Autodesk Inventor part; units mm, degrees
ref_plane "YZ Plane" through (0, 0, 0) normal (1, 0, 0) x (0, 1, 0)
ref_plane "XZ Plane" through (0, 0, 0) normal (0, 1, 0) x (-1, 0, 0)
ref_plane "XY Plane" through (0, 0, 0) normal (0, 0, 1) x (1, 0, 0)
sketch "Sketch1" plane through (0, 0, 0) normal (0, 0, 1) x (1, 0, 0)
  line L0 (-15.875, 29.0994) -> (-12.7, 29.0994) construction
  line L1 (-15.875, 51.3244) -> (-15.875, 29.0994) construction
  arc A0 (-9.525, 57.6744) -> (-15.875, 51.3244) centre (-9.525, 51.3244) ccw construction
  line L2 (9.525, 57.6744) -> (-9.525, 57.6744) construction
  arc A1 (15.875, 51.3244) -> (9.525, 57.6744) centre (9.525, 51.3244) ccw construction
  line L3 (15.875, 29.0994) -> (15.875, 51.3244) construction
  line L4 (12.7, 29.0994) -> (15.875, 29.0994) construction
  line L5 (12.7, 51.3244) -> (12.7, 29.0994) construction
  arc A2 (12.7, 51.3244) -> (9.525, 54.4994) centre (9.525, 51.3244) ccw construction
  line L6 (-9.525, 54.4994) -> (9.525, 54.4994) construction
  arc A3 (-9.525, 54.4994) -> (-12.7, 51.3244) centre (-9.525, 51.3244) ccw construction
  line L7 (-12.7, 29.0994) -> (-12.7, 51.3244) construction
  line L8 (-30.0912, 10.1284) -> (-15.5432, 53.35)
  line L9 (30.0912, 10.1284) -> (15.5432, 53.35)
  arc A4 (-9.525, 57.6744) -> (-15.5432, 53.35) centre (-9.525, 51.3244) ccw
  arc A5 (15.5432, 53.35) -> (9.525, 57.6744) centre (9.525, 51.3244) ccw
  line L10 (-9.525, 57.6744) -> (9.525, 57.6744)
  arc A6 (-30.0912, 10.1284) -> (30.0912, 10.1284) centre (0, 0) ccw
  line L11 (-17.9505, 54.1603) -> (-32.4985, 10.9386)
  arc A7 (-32.4985, 10.9386) -> (32.4985, 10.9386) centre (0, 0) ccw
  line L12 (32.4985, 10.9386) -> (17.9505, 54.1603)
  arc A8 (17.9505, 54.1603) -> (9.525, 60.2144) centre (9.525, 51.3244) ccw
  line L13 (9.525, 60.2144) -> (-9.525, 60.2144)
  arc A9 (-9.525, 60.2144) -> (-17.9505, 54.1603) centre (-9.525, 51.3244) ccw
  circle A10 centre (0, 0) radius 31.75 construction
  dimension "d0" = 2.54
extrude "Extrusion1" add sketch "Sketch1" along normal blind 9.297
properties part number "Weight Shifter Tension Strap 2" material "Rubber"
Build history of the part. All positions in model axes, mm. A direction names the side the tool comes from. Coordinates: 2 decimals unless noted, no trailing zeros. Order: outer loops, then holes, each group sorted by start corner. A loop starts at its lowest first (then second) coordinate and runs counter-clockwise, first axis right, second up. Notation, with made-up numbers: (-17.75, 39.25) - (-1.75, 39.25) arc R26 ccw to (-1.75, 73.25) - close; hole circle Ø6 at (17.5, 76). An arc over 180 degrees is marked (long way). Put each result on its own line as item: value.
1. Saw through at A-A (x = 0). Write the cut outline in (y, z), and give its area (3 significant figures).
Answer sheet:
outline: (-34.29, 0) - (-31.75, 0) - (-31.75, 9.3) - (-34.29, 9.3) - close; (57.67, 0) - (60.21, 0) - (60.21, 9.3) - (57.67, 9.3) - close
area: 47.2 mm^2
2. Drop flat-ended pins along their axis: P1, Ø1.5, axis at y = 38.5, z = 8.5, coming from the +X side; P2, Ø10, axis at x = 9.5, y = -21.5, coming from the +Z side; P3, Ø5, axis at x = -14, z = 5.5, coming from the -Y side; P4, Ø4, axis at y = 3, z = 6, coming from the -X side. Give the stop position or say it passes through.
Answer sheet:
P1: stops at x = 23.47
P2: passes through
P3: stops at y = -32.3
P4: stops at x = -34.28
3. Saw through at C-C (y = 0). Write the cut outline in (x, z), and give its area (3 significant figures).
Answer sheet:
outline: (-34.29, 0) - (-31.75, 0) - (-31.75, 9.3) - (-34.29, 9.3) - close; (31.75, 0) - (34.29, 0) - (34.29, 9.3) - (31.75, 9.3) - close
area: 47.2 mm^2
4. Probe line 1 along X through (y, z) = (0, 4); line 2 along Y through (x, z) = (0, 6.5); line 3 along Y through (x, z) = (-7.5, 0.5). List the from-to ranges inside material, lowest first. Write a range as [from, to].
Answer sheet:
line 1: x = [-34.29, -31.75], [31.75, 34.29]
line 2: y = [-34.29, -31.75], [57.67, 60.21]
line 3: y = [-33.46, -30.85], [57.67, 60.21]
5. Pull direction X, two halves, no side cores. Call faces 3 (the face through (-26, 24, 0)), 4 (the face through (13.19, 56.51, 4.58)), 5 (the face through (0.91, -34.278, 4.583)): pulls with the +X half, pulls with the -X half, needs draft (parallel to the pull), parting line crosses it, or undercut.
Answer sheet:
face 3: needs draft
face 4: undercut
face 5: parting line crosses it
6. Tool access for faces 1 (the face through (25.326, 32.247, 4.583)), 2 (the face through (22.92, 31.44, 4.58)): list every direction of +Z, -Z, +X, -X, +Y, -Y with a clear straight run to the whole face (end or side of a thin tool).
Answer sheet:
face 1: +Z, -Z, +X, +Y
face 2: +Z, -Z
